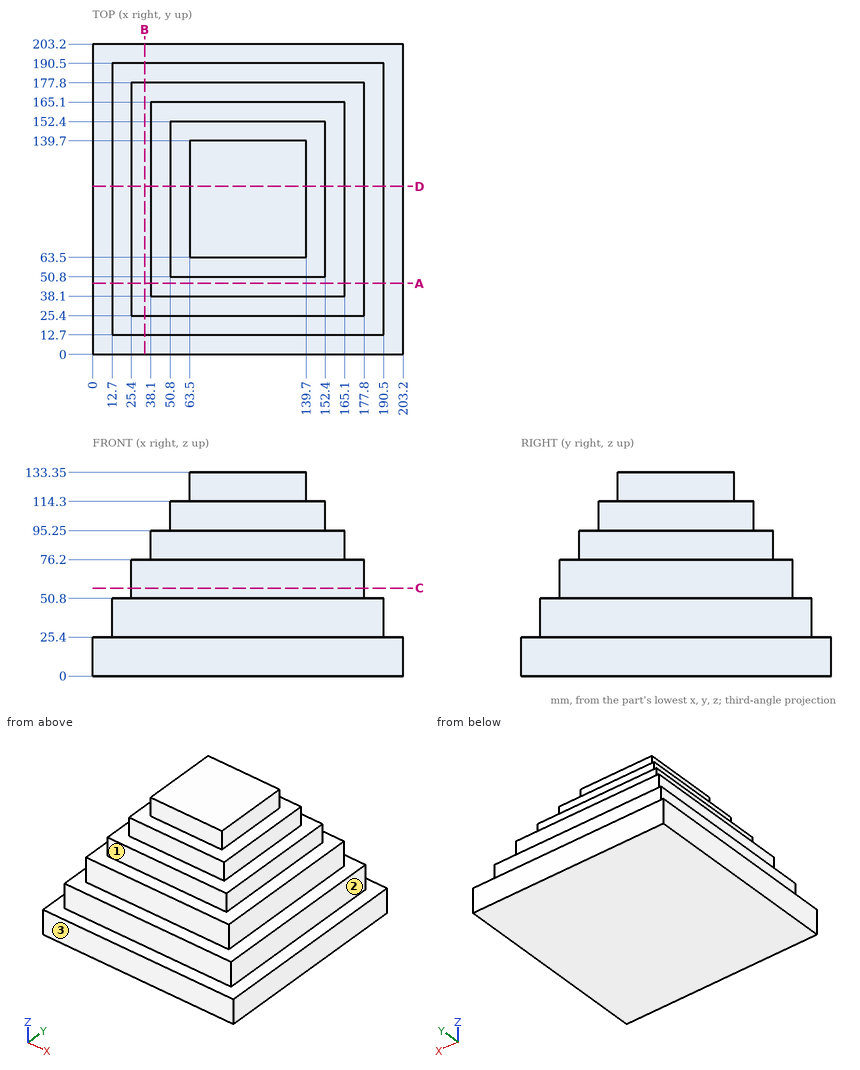
Could you check a few things on this drawing? It's one solid part, dimensions in mm from its lowest x, y, z. A direction names the side the tool comes from. Coordinates: 2 decimals unless noted, no trailing zeros. Order: outer loops, then holes, each group sorted by start corner. A loop starts at its lowest first (then second) coordinate and runs counter-clockwise, first axis right, second up.
1) Imagine slicing it at C-C on z = 57.5. List the corners of the cut face in (x, y) for me, and give its area (3 significant figures).
2) Which directions (+Z, -Z, +X, -X, +Y, -Y) give clear straight access to the entire face, cutting with the end or side of a thin tool? Please do the marked faces 1, 2 and 3.
3) Imagine slicing it at B-B on x = 34. List the corners of the cut face in (y, z) for me, and give its area (3 significant figures).
4) I need wall thicknesses on line 1 (Z direction, x = 40, y = 152); line 2 (Y direction, x = 122.5, z = 119); line 3 (X direction, y = 156.5, z = 29). Which ranges of each line are inside material? Lowest first, please.
5) Will these pins go through, and if not, where does the flat tip stop? pin 1 (1 mm diameter, centred on x = 37, z = 32.5, fed in from -Y); pin 2 (5.5 mm diameter, centred on y = 99, z = 100, fed in from -X); pin 3 (12.5 mm diameter, centred on x = 121, z = 65.5, fed in from +Y).
6) Imagine slicing it at D-D on y = 110. List the corners of the cut face in (x, z) for me.
7) Imagine slicing it at A-A on y = 46.5. List the corners of the cut face in (x, z) for me, and give its area (3 significant figures).
Response values:
1. outline: (25.4, 25.4) - (177.8, 25.4) - (177.8, 177.8) - (25.4, 177.8) - close
1. area: 23,200 mm2
2. face 1: +Z, +X, -X, -Y
2. face 2: +Z, +X, +Y, -Y
2. face 3: +Z, -Z, +X, -X, -Y
3. outline: (0, 0) - (203.2, 0) - (203.2, 25.4) - (190.5, 25.4) - (190.5, 50.8) - (177.8, 50.8) - (177.8, 76.2) - (25.4, 76.2) - (25.4, 50.8) - (12.7, 50.8) - (12.7, 25.4) - (0, 25.4) - close
3. area: 13,500 mm2
4. line 1: z = 0 to 95.25
4. line 2: y = 63.5 to 139.7
4. line 3: x = 12.7 to 190.5
5. pin 1: stops at y = 12.7
5. pin 2: stops at x = 50.8
5. pin 3: stops at y = 177.8
6. outline: (0, 0) - (203.2, 0) - (203.2, 25.4) - (190.5, 25.4) - (190.5, 50.8) - (177.8, 50.8) - (177.8, 76.2) - (165.1, 76.2) - (165.1, 95.25) - (152.4, 95.25) - (152.4, 114.3) - (139.7, 114.3) - (139.7, 133.35) - (63.5, 133.35) - (63.5, 114.3) - (50.8, 114.3) - (50.8, 95.25) - (38.1, 95.25) - (38.1, 76.2) - (25.4, 76.2) - (25.4, 50.8) - (12.7, 50.8) - (12.7, 25.4) - (0, 25.4) - close
7. outline: (0, 0) - (203.2, 0) - (203.2, 25.4) - (190.5, 25.4) - (190.5, 50.8) - (177.8, 50.8) - (177.8, 76.2) - (165.1, 76.2) - (165.1, 95.25) - (38.1, 95.25) - (38.1, 76.2) - (25.4, 76.2) - (25.4, 50.8) - (12.7, 50.8) - (12.7, 25.4) - (0, 25.4) - close
7. area: 16,000 mm2
